The listing builds one solid part. Answer for the finished solid, in the listing's coordinates (mm). Coordinates: 2 decimals unless noted, no trailing zeros. Write each loop counter-clockwise with the first axis right and the second up, starting at its lowest first coordinate (ties: lowest second). Pieces come first, ordered by that corner, then holes.
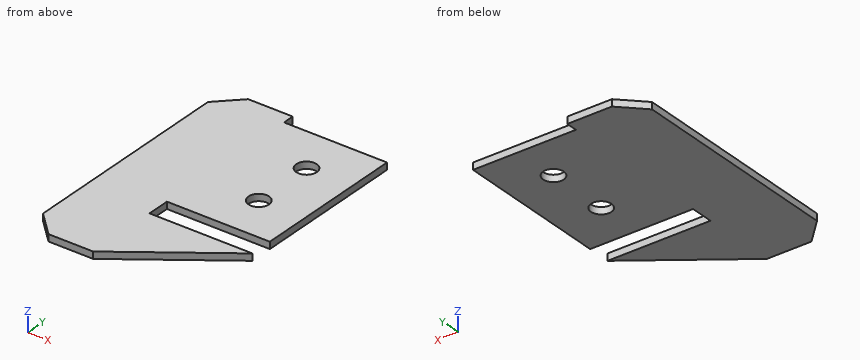
Autodesk Fusion 360 part; units mm, degrees
sketch "スケッチ1" plane through (0, 0, 0) normal (0, 0, 1) x (1, 0, 0)
  line L0 (-15.5, 115) -> (-74.5, 115)
  line L1 (-74.5, 115) -> (-74.5, -115)
  line L2 (-74.5, -115) -> (-15.5, -115)
  line L3 (74.5, -30) -> (74.5, 105)
  line L4 (68.0217, 105) -> (-74.5, -115) construction
  line L5 (-74.5, 115) -> (45.8131, -70.7183) construction
  line L6 (-15.5, 115) -> (-15.5, 105)
  line L7 (-15.5, 105) -> (74.5, 105)
  line L8 (-74.5, -115) -> (-15.5, -115) construction
  line L9 (74.5, -50) -> (-15.5, -115)
  line L10 (74.5, -50) -> (-15.5, -50)
  line L11 (-15.5, -50) -> (-15.5, -30)
  line L12 (-15.5, -30) -> (74.5, -30)
  dimension "d2" = 230
  dimension "d5" = 59
  dimension "d7" = 90
  dimension "d8" = 20
extrude "押し出し1" add sketch "スケッチ1" along normal blind 6
chamfer "面取り1" distance 20 angle 45 2 edges at (-74.5, -115, 3) (-74.5, 115, 3)
sketch "スケッチ2" plane through (0, 0, 6) normal (0, 0, 1) x (-1, 0, 0)
  line L0 (54.5, -115) -> (74.5, -95)
  line L1 (74.5, -95) -> (74.5, 95)
  line L2 (74.5, 95) -> (54.5, 115)
  line L3 (54.5, 115) -> (15.5, 115)
  line L4 (15.5, 115) -> (-74.5, 50)
  line L5 (-74.5, 50) -> (15.5, 50)
  line L6 (15.5, 50) -> (15.5, 30)
  line L7 (15.5, 30) -> (-74.5, 30)
  line L8 (-74.5, 30) -> (-74.5, -105)
  line L9 (-74.5, -105) -> (15.5, -105)
  line L10 (15.5, -105) -> (15.5, -115)
  line L11 (15.5, -115) -> (54.5, -115)
  line L12 (-74.5, -105) -> (-34.5, -105) construction
  line L13 (-34.5, -105) -> (-34.5, -65) construction
  line L14 (-34.5, -65) -> (-74.5, -65) construction
  line L15 (-74.5, -65) -> (-74.5, -105) construction
  line L16 (-34.5, -65) -> (-34.5, -10) construction
  point P0 (-34.5, -65)
  point P1 (-34.5, -10)
  dimension "d12" = 40
  dimension "d13" = 40
  dimension "d14" = 55
hole "穴1" at (34.5, 65, 6) at (34.5, 10, 6) direction (0, 0, -1) diameter 18 end through all
equation "d5 = 20 mm + 39 mm"
1. Find the intervals of material crossed by L1, parallel to X at y = 10, z = 2.3; L2, parallel to Y at x = 34.5, z = 4.75; L3, parallel to Y at x = 45, z = 0.9, in increasing order.
Results found:
L1: x = -74.5 to 25.5, 43.5 to 74.5
L2: y = -78.89 to -50, -30 to 1, 19 to 56, 74 to 105
L3: y = -71.31 to -50, -30 to 105
2. Section B-B on z = 2.9 is taken. Give the vertices of the cut face in (x, y), then the cut area to 3 significant figures.
Results found:
outline: (-74.5, -95) - (-54.5, -115) - (-15.5, -115) - (74.5, -50) - (-15.5, -50) - (-15.5, -30) - (74.5, -30) - (74.5, 105) - (-15.5, 105) - (-15.5, 115) - (-54.5, 115) - (-74.5, 95) - close; hole circle Ø18 at (34.5, 10); hole circle Ø18 at (34.5, 65)
area: 27,700 mm2
3. Flat-ended cylindrical pins translate along their axes: P1, Ø11, axis at x = 34.5, y = 10, coming from the +Z side; P2, Ø1.8, axis at x = 23, z = 3, coming from the -Y side; P3, Ø2, axis at y = -64, z = 5, coming from the +X side; P4, Ø3, axis at y = -43.5, z = 3, coming from the +X side. Find the tip coordinate at first contact, or state that the pin passes through.
Results found:
P1: passes through
P2: stops at y = -87.84
P3: stops at x = 56.5
P4: stops at x = -15.5
4. Section C-C on x = 34.5 is taken. Give the vertices of the cut face in (y, z), then the cut area to 3 significant figures.
Results found:
outline: (-78.89, 0) - (-50, 0) - (-50, 6) - (-78.89, 6) - close; (-30, 0) - (1, 0) - (1, 6) - (-30, 6) - close; (19, 0) - (56, 0) - (56, 6) - (19, 6) - close; (74, 0) - (105, 0) - (105, 6) - (74, 6) - close
area: 767 mm2
5. Section A-A on y = 65 is taken. Give the vertices of the cut face in (x, z).
Results found:
outline: (-74.5, 0) - (25.5, 0) - (25.5, 6) - (-74.5, 6) - close; (43.5, 0) - (74.5, 0) - (74.5, 6) - (43.5, 6) - close
6. Section D-D on y = -75 is taken. Give the vertices of the cut face in (x, z).
Results found:
outline: (-74.5, 0) - (39.88, 0) - (39.88, 6) - (-74.5, 6) - close
